from build123d import *

# Parameters (mm, degrees)
SKETCH1_R           = 6.5151
BOSS_EXTRUDE1_DEPTH = 3.3676
BOSS_EXTRUDE2_DEPTH = 2.5146
BOSS_EXTRUDE3_DEPTH = 0.03175
BOSS_EXTRUDE4_DEPTH = 0.2032
BOSS_EXTRUDE5_DEPTH = 0.2032
BOSS_EXTRUDE6_DEPTH = 0.2032
BOSS_EXTRUDE7_DEPTH = 0.2032


with BuildPart() as part:
    # Sketch1 → Boss-Extrude1 (new body)
    with BuildSketch(Plane(origin=(0, 10.383607632, 0), x_dir=(-1, 0, 0), z_dir=(0, -1, 0))):
        with Locations((-86.1568, 0.188358884)):
            Circle(SKETCH1_R)
    extrude(amount=BOSS_EXTRUDE1_DEPTH)

    # Sketch2 → Boss-Extrude2 (add)
    with BuildSketch(Plane(origin=(0, 7.869007632, 0), x_dir=(1, 0, 0), z_dir=(0, 1, 0))):
        with BuildLine():
            Line((83.562463772, 6.164640968), (79.993269461, 4.615234502))
            ThreePointArc((79.993269461, 4.615234502), (77.089, 0.188358884), (79.993269461, -4.238516734))
            Line((79.993269461, -4.238516734), (83.562463772, -5.7879232))
            ThreePointArc((83.562463772, -5.7879232), (92.6719, 0.188358884), (83.562463772, 6.164640968))
        make_face()
    extrude(amount=BOSS_EXTRUDE2_DEPTH)

    # Sketch3 → Boss-Extrude3 (add)
    with BuildSketch(Plane(origin=(0, 10.415357632, 0), x_dir=(1, 0, 0), z_dir=(0, 1, 0))):
        with BuildLine():
            Line((86.379362148, 2.834929745), (86.331172499, 2.813512123))
            ThreePointArc((86.331172499, 2.813512123), (87.57388973, 2.642364143), (88.826675515, 2.706905023))
            ThreePointArc((88.826675515, 2.706905023), (88.743147222, -0.307968876), (87.717246323, -3.144158035))
            ThreePointArc((87.717246323, -3.144158035), (85.599615489, -1.990016157), (83.209989222, -1.664301363))
            ThreePointArc((83.209989222, -1.664301363), (83.226670097, -2.157743319), (83.268922831, -2.649655834))
            ThreePointArc((83.268922831, -2.649655834), (83.013982099, -2.96896843), (82.694669503, -2.714027698))
            ThreePointArc((82.694669503, -2.714027698), (82.970684724, 1.003656964), (84.577363687, 4.367575269))
            ThreePointArc((84.577363687, 4.367575269), (84.981125023, 4.430281687), (85.043831441, 4.026520351))
            ThreePointArc((85.043831441, 4.026520351), (84.845175329, 3.744205128), (84.656890151, 3.45486998))
            ThreePointArc((84.656890151, 3.45486998), (85.187045427, 3.19462014), (85.738141542, 2.982281574))
            ThreePointArc((85.738141542, 2.982281574), (85.741341744, 2.997904944), (85.745516089, 3.013296689))
            ThreePointArc((85.745516089, 3.013296689), (85.213902251, 3.217551458), (84.701749715, 3.466615834))
            ThreePointArc((84.701749715, 3.466615834), (84.880937437, 3.740370401), (85.069461538, 4.00778107))
            ThreePointArc((85.069461538, 4.00778107), (84.999864331, 4.455911764), (84.551733629, 4.386314602))
            ThreePointArc((84.551733629, 4.386314602), (82.940000597, 1.01181459), (82.663117122, -2.717564614))
            ThreePointArc((82.663117122, -2.717564614), (83.017519015, -3.000520811), (83.300475212, -2.646118918))
            ThreePointArc((83.300475212, -2.646118918), (83.259289868, -2.171130031), (83.242027928, -1.694671533))
            ThreePointArc((83.242027928, -1.694671533), (85.576128395, -2.015738406), (87.651108795, -3.131787359))
            ThreePointArc((87.651108795, -3.131787359), (87.69360158, -3.153679255), (87.735992687, -3.175767397))
            ThreePointArc((87.735992687, -3.175767397), (88.775617442, -0.307140697), (88.853849034, 2.743059067))
            ThreePointArc((88.853849034, 2.743059067), (87.612284437, 2.672606475), (86.379362148, 2.834929745))
        make_face()
    extrude(amount=-BOSS_EXTRUDE3_DEPTH)

    # Sketch4 → Boss-Extrude4 (add)
    with BuildSketch(Plane(origin=(0, 10.383607632, 0), x_dir=(1, 0, 0), z_dir=(0, 1, 0))):
        with BuildLine():
            Line((87.971211641, 4.006634675), (86.091611641, 4.842012453))
            ThreePointArc((86.091611641, 4.842012453), (85.756344283, 4.713063514), (85.8852933, 4.377796186))
            Line((85.8852933, 4.377796186), (86.1568, 4.257126542))
            Line((86.1568, 4.257126542), (86.1568, 3.291926542))
            Line((86.1568, 3.291926542), (85.8852933, 3.171256897))
            ThreePointArc((85.8852933, 3.171256897), (85.756344337, 2.835989594), (86.091611641, 2.707040631))
            Line((86.091611641, 2.707040631), (87.971211641, 3.542418409))
            ThreePointArc((87.971211641, 3.542418409), (88.12205247, 3.774526542), (87.971211641, 4.006634675))
        make_face()
        Polygon((87.24265, 3.774526542), (86.614, 4.053926542), (86.614, 3.495126542), align=None, mode=Mode.SUBTRACT)
    extrude(amount=BOSS_EXTRUDE4_DEPTH)

    # Sketch5 → Boss-Extrude5 (add)
    with BuildSketch(Plane(origin=(0, 10.383607632, 0), x_dir=(1, 0, 0), z_dir=(0, 1, 0))):
        with BuildLine():
            Line((88.12205247, 0.447338975), (88.12205247, 1.988743646))
            ThreePointArc((88.12205247, 1.988743646), (87.980866694, 2.216315505), (87.714265455, 2.19089595))
            Line((87.714265455, 2.19089595), (86.24245247, 1.071216772))
            Line((86.24245247, 1.071216772), (86.24245247, 1.988743646))
            ThreePointArc((86.24245247, 1.988743646), (85.98845247, 2.242743706), (85.73445247, 1.988743646))
            Line((85.73445247, 1.988743646), (85.73445247, 0.495012101))
            ThreePointArc((85.73445247, 0.495012101), (85.875638247, 0.267440242), (86.142239485, 0.292859797))
            Line((86.142239485, 0.292859797), (87.61405247, 1.412538975))
            Line((87.61405247, 1.412538975), (87.61405247, 0.447338975))
            ThreePointArc((87.61405247, 0.447338975), (87.86805247, 0.193338975), (88.12205247, 0.447338975))
        make_face()
    extrude(amount=BOSS_EXTRUDE5_DEPTH)

    # Sketch6 → Boss-Extrude6 (add)
    with BuildSketch(Plane(origin=(0, 10.383607632, 0), x_dir=(1, 0, 0), z_dir=(0, 1, 0))):
        with BuildLine():
            Line((88.12205247, -2.20349139), (88.12205247, -0.573641116))
            ThreePointArc((88.12205247, -0.573641116), (88.022972158, -0.372355522), (87.803029713, -0.328104884))
            ThreePointArc((87.803029713, -0.328104884), (86.82154331, -0.641121728), (85.876084624, -1.050270813))
            ThreePointArc((85.876084624, -1.050270813), (85.745367006, -1.204405708), (85.76854522, -1.405172817))
            ThreePointArc((85.76854522, -1.405172817), (86.002778478, -1.790740386), (86.25361081, -2.165721333))
            ThreePointArc((86.25361081, -2.165721333), (86.607396093, -2.227914435), (86.669589172, -1.874129148))
            ThreePointArc((86.669589172, -1.874129148), (86.505953581, -1.633172635), (86.349528836, -1.387473738))
            ThreePointArc((86.349528836, -1.387473738), (86.973563185, -1.12669528), (87.61405247, -0.909444852))
            Line((87.61405247, -0.909444852), (87.61405247, -2.20349139))
            ThreePointArc((87.61405247, -2.20349139), (87.86805247, -2.45749139), (88.12205247, -2.20349139))
        make_face()
    extrude(amount=BOSS_EXTRUDE6_DEPTH)

    # Sketch7 → Boss-Extrude7 (add)
    with BuildSketch(Plane(origin=(0, 10.383607632, 0), x_dir=(1, 0, 0), z_dir=(0, 1, 0))):
        with BuildLine():
            Line((85.73445247, -2.721325206), (85.73445247, -4.351175481))
            ThreePointArc((85.73445247, -4.351175481), (85.838455656, -4.55615586), (86.065294641, -4.593273149))
            ThreePointArc((86.065294641, -4.593273149), (87.050038854, -4.224609495), (87.992239729, -3.75782093))
            ThreePointArc((87.992239729, -3.75782093), (88.12205247, -3.536250363), (87.992239763, -3.314679777))
            ThreePointArc((87.992239763, -3.314679777), (87.050038872, -2.8478912), (86.065294641, -2.479227539))
            ThreePointArc((86.065294641, -2.479227539), (85.838455656, -2.516344828), (85.73445247, -2.721325206))
        make_face()
        with BuildLine():
            Line((86.1822, -3.053650344), (86.1822, -4.018850344))
            ThreePointArc((86.1822, -4.018850344), (86.761323847, -3.795601976), (87.325204148, -3.536250344))
            ThreePointArc((87.325204148, -3.536250344), (86.761323847, -3.276898711), (86.1822, -3.053650344))
        make_face(mode=Mode.SUBTRACT)
    extrude(amount=BOSS_EXTRUDE7_DEPTH)


solid = part.part
Design review of the part built by this model. Coordinates are the model's own, in mm. A direction names the side the tool comes from. Round coordinates to 2 decimals unless told otherwise and drop trailing zeros. Loops run counter-clockwise (first coordinate to the right, second up) from the corner with the lowest first, then second, coordinate; pieces in that order, holes last. Notation, with made-up numbers: (36, 12.5) - (73, 12.5) arc R9 ccw to (73, 22.5) - close; hole circle Ø6 at (-35, -11). An arc over 180 degrees is marked (long way). One line per item, written item: value. Start each with the question number.
1) Consider section C-C on y = 8.25. Give the boundary of the cut face in (x, z) (3 decimals).
2) Draft analysis for pull direction X (two halves, no side actions). For faces 3 (the cylindrical face through (77.09, 9.11, -0.27)), 4 (the flat face through (86, 7.016, 0)), 5 (the flat face through (86.6, 10.384, 3.5)), state which applies: +X half, -X half, draft (parallel to the pull), parting line (faces both ways), or undercut.
3) Insertion check: pin 1 Ø1 at (x, y) = (78.5, 10) entering from +Z; pin 2 Ø4 at (x, z) = (78.5, -0.5) entering from +Y; pin 3 Ø1 at (x, y) = (89.5, 8.5) entering from -Z. Each pin has a flat end and moves straight along its axis. Give the tip position at first contact, or say it passes through.
4) To check wall thickness, follow L1, parallel to Y at x = 82.5, z = -0.5; L2, parallel to X at y = 8.65, z = 0; L3, parallel to X at y = 7.3, z = 3.5. State the ranges of each line that lie inside material, in increasing order. Write a range as from..to.
5) For faces 1 (the flat face through (86.9, 10.587, -1.2)), 2 (the flat face through (85, 10.384, 3)), list the 3-axis set-ups (+Z, -Z, +X, -X, +Y, -Y) from which the entire face can be reached by the end or side of a thin tool; tool diameter is ignored.
Reported:
1. outline: (79.993, -4.615) - (83.562, -6.165) arc R6.515 ccw (long way) to (83.562, 5.788) - (79.993, 4.239) arc R4.826 ccw to start
2. face 3: -X half
2. face 4: draft
2. face 5: undercut
3. pin 1: stops at z = 3.66
3. pin 2: stops at y = 10.38
3. pin 3: stops at z = -6.05
4. L1: y = 7.02..10.38
4. L2: x = 77.09..92.67
4. L3: x = 80.79..91.53
5. face 1: +Z, -Z, +X, -X, +Y
5. face 2: +Y
